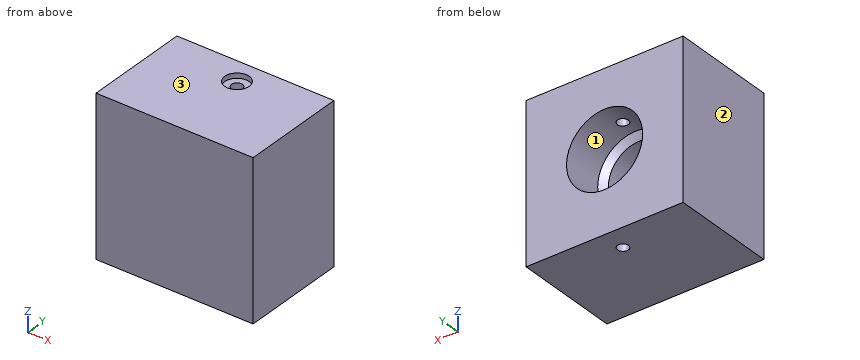
from build123d import *

# Parameters (mm, degrees)
SKETCH2_W                                           = 25.4
SKETCH2_H                                           = 17.146948585
BOSS_EXTRUDE1_DEPTH                                 = 12.7
F_7_16_20_TAPPED_HOLE1_D                            = 9.92124
F_7_16_20_TAPPED_HOLE1_DEPTH                        = 12.235907381
F_7_16_20_TAPPED_HOLE1_TIP                          = 2.980641204
F_7_16_CLEARANCE_HOLE3_D                            = 12.30376
F_7_16_CLEARANCE_HOLE3_DEPTH                        = 6.604
F_7_16_CLEARANCE_HOLE3_TIP                          = 3.696422425
CBORE_FOR_0_BINDING_HEAD_MACHINE_SCREW1_D           = 1.778
CBORE_FOR_0_BINDING_HEAD_MACHINE_SCREW1_CBORE_D     = 3.97002
CBORE_FOR_0_BINDING_HEAD_MACHINE_SCREW1_CBORE_DEPTH = 0.8128


with BuildPart() as part:
    # Sketch2 → Boss-Extrude1 (new, symmetric)
    with BuildSketch(Plane(origin=(0, 0, 0), x_dir=(0, 0, -1), z_dir=(1, 0, 0))):
        with Locations((0.311038218, -8.573474293)):
            Rectangle(SKETCH2_W, SKETCH2_H)
    extrude(amount=BOSS_EXTRUDE1_DEPTH, both=True)

    # 7/16-20 Tapped Hole1
    with Locations(Plane(origin=(0, 0, 0), x_dir=(1, 0, 0), z_dir=(0, 1, 0))):
        with Locations((0, 0)):
            Hole(F_7_16_20_TAPPED_HOLE1_D / 2, depth=F_7_16_20_TAPPED_HOLE1_DEPTH)
            with Locations((0, 0, -(F_7_16_20_TAPPED_HOLE1_DEPTH + F_7_16_20_TAPPED_HOLE1_TIP / 2))):  # 118° drill point
                Cone(0, F_7_16_20_TAPPED_HOLE1_D / 2, F_7_16_20_TAPPED_HOLE1_TIP, mode=Mode.SUBTRACT)

    # 7/16 Clearance Hole3
    with Locations(Plane(origin=(0, 0, 0), x_dir=(1, 0, 0), z_dir=(0, 1, 0))):
        with Locations((0, 0)):
            Hole(F_7_16_CLEARANCE_HOLE3_D / 2, depth=F_7_16_CLEARANCE_HOLE3_DEPTH)
            with Locations((0, 0, -(F_7_16_CLEARANCE_HOLE3_DEPTH + F_7_16_CLEARANCE_HOLE3_TIP / 2))):  # 118° drill point
                Cone(0, F_7_16_CLEARANCE_HOLE3_D / 2, F_7_16_CLEARANCE_HOLE3_TIP, mode=Mode.SUBTRACT)

    # CBORE for #0 Binding Head Machine Screw1 (through all)
    with Locations(Plane(origin=(0, -3.914304801, 12.388961782), x_dir=(1, 0, 0), z_dir=(0, 0, 1))):
        with Locations((0, 0)):
            CounterBoreHole(CBORE_FOR_0_BINDING_HEAD_MACHINE_SCREW1_D / 2, CBORE_FOR_0_BINDING_HEAD_MACHINE_SCREW1_CBORE_D / 2, CBORE_FOR_0_BINDING_HEAD_MACHINE_SCREW1_CBORE_DEPTH)


solid = part.part
Design review of the part built by this model. Coordinates are the model's own, in mm. Face numbers are marked on the shaded views. Coordinates: 2 decimals unless noted, no trailing zeros. Order: outer loops, then holes, each group sorted by start corner. A loop starts at its lowest first (then second) coordinate and runs counter-clockwise, first axis right, second up. Notation, with made-up numbers: (34.25, 38.25) -> (92.25, 38.25) arc R24 cw to (92.25, 68.25) -> close; hole circle Ø3 at (87.5, 88). An arc over 180 degrees is marked (long way). Use one line per item in the form item = value. Start each with the question number.
(1) The part is to be moulded in two halves that separate along Z. For the marked faces 1, 2 and 3, say which applies: +Z half, -Z half, draft (parallel to the pull), parting line (faces both ways), or undercut.
(2) For probe 1 along Z at (x, y) = (0, -6.25); probe 2 along Y at (x, z) = (0, 7.5); probe 3 along X at (y, z) = (-10.25, 1.75), list the stretches that pass through material, from the lowest coordinate up.
(3) Insertion check: pin 1 (7.5 mm diameter, centred on x = 0, z = 0, fed in from +Y); pin 2 (1.4 mm diameter, centred on x = 0, y = -3.91, fed in from +Z). Each pin has a flat end and moves straight along its axis. Give the tip position at first contact, or say it passes through.
(4) Add section B-B on x = 0.5. Give the number of separate pieces and of enclosed holes in the cut face, plus the area to 3 significant figures.
(5) Add section C-C on y = -10.5. State the section outline as (x, z) points, plus the area to 3 significant figures.
(6) Add section A-A on y = -6.25. State the section outline as (x, z) points.
Answer block:
q1.face_1 = undercut
q1.face_2 = draft
q1.face_3 = +Z half
q2.probe_1 = -13.01 to -6.15, 6.15 to 12.39
q2.probe_2 = -17.15 to -4.8, -3.03 to 0
q2.probe_3 = -12.7 to -4.64, 4.64 to 12.7
q3.pin_1 = -12.96
q3.pin_2 = through
q4.separate_pieces = 3
q4.enclosed_holes = 0
q4.area = 263 mm²
q5.outline = (-12.7, -13.01) -> (12.7, -13.01) -> (12.7, 12.39) -> (-12.7, 12.39) -> close; hole circle Ø9.92 at (0, 0)
q5.area = 568 mm²
q6.outline = (-12.7, -13.01) -> (12.7, -13.01) -> (12.7, 12.39) -> (-12.7, 12.39) -> close; hole circle Ø12.3 at (0, 0)
